Could you check a few things on this model? Use its own coordinates, in mm. A direction names the side the tool comes from. Round coordinates to 2 decimals unless told otherwise and drop trailing zeros. Write each loop counter-clockwise with the first axis right and the second up, starting at its lowest first coordinate (ties: lowest second). Pieces come first, ordered by that corner, then holes. Notation, with made-up numbers: (69.5, 40.25) -> (76.5, 40.25) arc R23 cw to (76.5, 75.25) -> close; hole circle Ø5 at (26, 37). An arc over 180 degrees is marked (long way). Answer in a Markdown table with one row per item. Add a question column.
```python
from build123d import *

# Parameters (mm, degrees)
BOSS_EXTRUDE1_DEPTH       = 19.05
SKETCH2_W                 = 390
SKETCH2_H                 = 47
SKETCH2_H_2               = 16
CUT_EXTRUDE2_DEPTH        = 4.05
M6_CLEARANCE_HOLE1_D      = 6.6
M6_CLEARANCE_HOLE2_D      = 6.6
M3X0_5_TAPPED_HOLE1_D     = 2.5
M3X0_5_TAPPED_HOLE1_DEPTH = 7.5
M3X0_5_TAPPED_HOLE1_TIP   = 0.751075774
M8X1_0_TAPPED_HOLE1_D     = 7
M8_CLEARANCE_HOLE1_D      = 9
FILLET1_R                 = 10
CHAMFER1_SIZE             = 1


with BuildPart() as part:
    # Sketch1 → Boss-Extrude1 (new body)
    with BuildSketch(Plane.XY):
        Polygon((-195, 50), (-195, -25), (195, -25), (195, 200), (115, 200), (115, 160), align=None)
    extrude(amount=BOSS_EXTRUDE1_DEPTH)

    # Sketch2 → Cut-Extrude2 (cut)
    with BuildSketch(Plane(origin=(0, 0, 0), x_dir=(-1, 0, 0), z_dir=(0, 0, -1))):
        with Locations((0, -1.5)):
            Rectangle(SKETCH2_W, SKETCH2_H)
        with Locations((0, 40.5)):
            Rectangle(SKETCH2_W, SKETCH2_H_2)
    extrude(amount=-CUT_EXTRUDE2_DEPTH, mode=Mode.SUBTRACT)

    # M6 Clearance Hole1 (through all)
    with Locations(Plane(origin=(0, 0, 4.05), x_dir=(-1, 0, 0), z_dir=(0, 0, -1))):
        with Locations((127, 16), (163, 16), (163, -16), (127, -16)):
            Hole(M6_CLEARANCE_HOLE1_D / 2)

    # M6 Clearance Hole2 (through all)
    with Locations(Plane(origin=(0, 0, 4.05), x_dir=(-1, 0, 0), z_dir=(0, 0, -1))):
        with Locations((-163, 16), (-127, 16), (-127, -16), (-163, -16)):
            Hole(M6_CLEARANCE_HOLE2_D / 2)

    # M3x0.5 Tapped Hole1
    with Locations(Plane(origin=(0, 0, 4.05), x_dir=(-1, 0, 0), z_dir=(0, 0, -1))):
        with Locations((-180, 42.5), (-160, 42.5), (180, 42.5), (160, 42.5)):
            Hole(M3X0_5_TAPPED_HOLE1_D / 2, depth=M3X0_5_TAPPED_HOLE1_DEPTH)
            with Locations((0, 0, -(M3X0_5_TAPPED_HOLE1_DEPTH + M3X0_5_TAPPED_HOLE1_TIP / 2))):  # 118° drill point
                Cone(0, M3X0_5_TAPPED_HOLE1_D / 2, M3X0_5_TAPPED_HOLE1_TIP, mode=Mode.SUBTRACT)

    # M8x1.0 Tapped Hole1 (through all)
    with Locations(Plane(origin=(0, 0, 0), x_dir=(-1, 0, 0), z_dir=(0, 0, -1))):
        with Locations((-175, 190), (-135, 190), (-65, 126.666666667), (-175, 63.333333333), (-65, 0)):
            Hole(M8X1_0_TAPPED_HOLE1_D / 2)

    # M8 Clearance Hole1 (through all)
    with Locations(Plane(origin=(0, 0, 0), x_dir=(-1, 0, 0), z_dir=(0, 0, -1))):
        with Locations((-22.6, 80), (17.4, 80)):
            Hole(M8_CLEARANCE_HOLE1_D / 2)

    # Fillet1
    fillet1_edges = [part.edges().sort_by_distance(p)[0] for p in [
        (115, 160, 9.525),
    ]]
    fillet(fillet1_edges, radius=FILLET1_R)

    # Chamfer1
    chamfer1_edges = [part.edges().sort_by_distance(p)[0] for p in [
        (115, 200, 9.525),
        (195, 200, 9.525),
        (195, -25, 11.55),
        (-195, -25, 11.55),
        (-195, 22, 2.025),
        (195, 22, 2.025),
        (-195, 32.5, 2.025),
        (-195, 48.5, 2.025),
        (195, 48.5, 2.025),
        (195, 32.5, 2.025),
    ]]
    chamfer(chamfer1_edges, length=CHAMFER1_SIZE)


solid = part.part
```
(1) Suppose I cut it at C-C, the plane x = 103. Please give me the cut outline in (y, z), then the cut area to 3 significant figures.
(2) For P1, Ø3, axis at x = -101.5, z = 7, coming from the +Y side; P2, Ø7.5, axis at x = -127, y = -16, coming from the -Z side; P3, Ø3, axis at x = -69.5, z = 2, coming from the -Y side, each with a flat end and sliding along its axis, tell me the tip position at first contact or that it passes through.
(3) I need wall thicknesses on L1, parallel to Y at x = 175, z = 15.25; L2, parallel to Y at x = 163, z = 16.25; L3, parallel to X at y = 42.5, z = 6. Which ranges of each line are inside material? Lowest first, please.
(4) Suppose I cut it at A-A, the plane z = 7.5. State how many separate pieces and enclosed holes the cut face has, then the cut area to 3 significant figures.
(5) Suppose I cut it at D-D, the plane y = 113. Please give me the cut outline in (x, z).
(6) Suppose I cut it at B-B, the plane x = -17.4. Please give me the cut outline in (y, z).
(7) If we mould it in two halves opening along X, with no side actions, what happens to faces 1 (the face through (61.503, 0.154, 11.655)), 2 (the face through (156, 200, 9)), 3 (the face through (113.1, 161.2, 9.7)), 4 (the face through (25.019, 83.794, 9.658))? For each: pulls with the +X half, pulls with the -X half, needs draft (parallel to the pull), parting line crosses it, or undercut.
(8) On a 3-axis mill with a long thin cutter (end or side, diameter ignored), from which of +Z, -Z, +X, -X, +Y, -Y can I reach the whole of each face in a straight line? I mean faces 5 (the face through (3, -1, 4.05)), 6 (the face through (115, 183, 9)), 7 (the face through (178.233, 188.659, 9.658)). Say none if no direction works.
Response:
| question | item | result |
|---|---|---|
| 1 | outline | (-25, 4.05) -> (22, 4.05) -> (22, 0) -> (32.5, 0) -> (32.5, 4.05) -> (48.5, 4.05) -> (48.5, 0) -> (155.74, 0) -> (155.74, 19.05) -> (-25, 19.05) -> close |
| 1 | area | 3,190 mm² |
| 2 | P1 | y = 83.71 |
| 2 | P2 | z = 4.05 |
| 2 | P3 | y = 22 |
| 3 | L1 | -25 to 59.83, 66.83 to 186.5, 193.5 to 200 |
| 3 | L2 | -25 to -19.3, -12.7 to 12.7, 19.3 to 200 |
| 3 | L3 | -195 to -181.25, -178.75 to -161.25, -158.75 to 158.75, 161.25 to 178.75, 181.25 to 195 |
| 4 | separate pieces | 1 |
| 4 | enclosed holes | 19 |
| 4 | area | 57,700 mm² |
| 5 | outline | (-17.45, 0) -> (195, 0) -> (195, 19.05) -> (-17.45, 19.05) -> close |
| 6 | outline | (-25, 4.05) -> (22, 4.05) -> (22, 0) -> (32.5, 0) -> (32.5, 4.05) -> (48.5, 4.05) -> (48.5, 0) -> (75.5, 0) -> (75.5, 19.05) -> (-25, 19.05) -> close; (84.5, 0) -> (113.02, 0) -> (113.02, 19.05) -> (84.5, 19.05) -> close |
| 7 | face 1 | undercut |
| 7 | face 2 | needs draft |
| 7 | face 3 | pulls with the -X half |
| 7 | face 4 | undercut |
| 8 | face 5 | -Z, +X, -X, -Y |
| 8 | face 6 | +Z, -Z, -X, +Y |
| 8 | face 7 | +Z, -Z |
